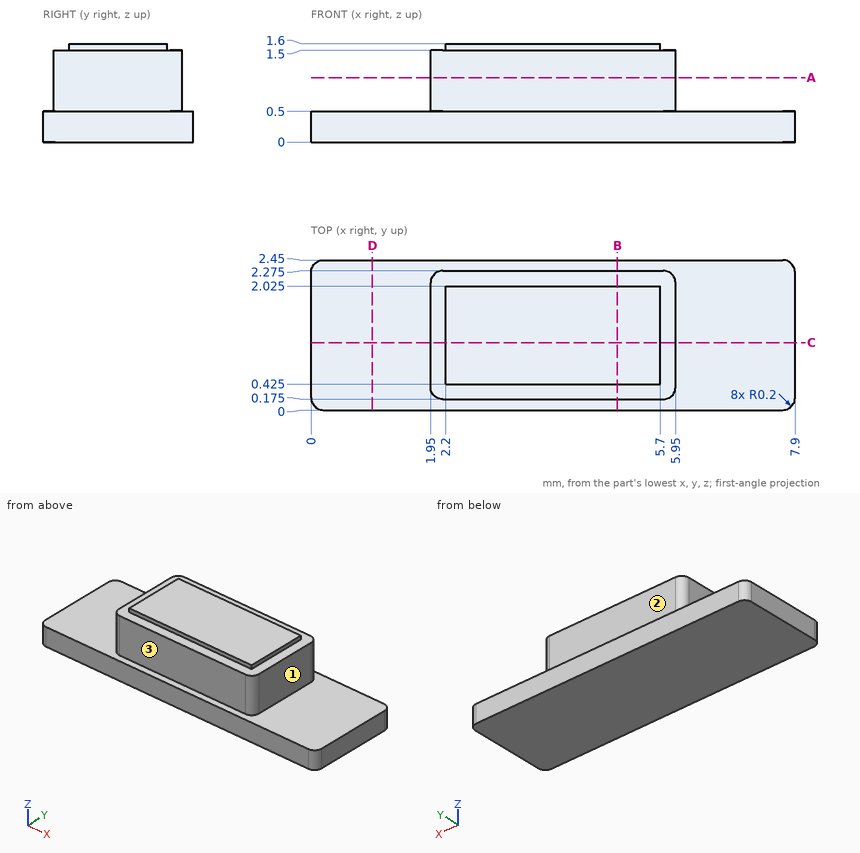
Input: dimensioned drawing with shaded views. Units: mm. Origin: part minimum x, y, z. A direction names the side the tool comes from. Round coordinates to 2 decimals unless told otherwise and drop trailing zeros. Order: outer loops, then holes, each group sorted by start corner. A loop starts at its lowest first (then second) coordinate and runs counter-clockwise, first axis right, second up. Notation, with made-up numbers: (24.25, 47) -> (34.25, 47) arc R33 ccw to (34.25, 78) -> close; hole circle Ø5 at (85.25, 19.5). An arc over 180 degrees is marked (long way). Put each result on its own line as item: value. Start each with the question number.
Q1. Section A-A on z = 1.05. Return the cut outline in (x, y) (3 decimals), and give its area (3 significant figures).
Q2. Line query: probe 1 along Z at (x, y) = (2, 1.35); probe 2 along Z at (x, y) = (7, 2); probe 3 along X at (y, z) = (0.55, 1.4). Output: solid intervals per line, ascending.
Q3. Reachability of the marked faces 1, 2 and 3 from +Z, -Z, +X, -X, +Y, -Y: full face, straight path, thin tool, end or side. Return the list, or none.
Q4. Section B-B on x = 5. Return the cut outline in (y, z) (3 decimals), and give its area (4 significant figures).
Q5. First-contact query: pin 1 (0.8 mm diameter, centred on x = 3, z = 1, fed in from -Y) (3 decimals); pin 2 (1 mm diameter, centred on x = 1, y = 1, fed in from +Z). Flat tips, straight axial feed; report the tip coordinate or a pass-through.
Q6. Section C-C on y = 1.1. Return the cut outline in (x, z).
Q7. Section D-D on x = 1. Return the cut outline in (y, z), and give its area (4 significant figures).
Ans:
1. outline: (1.95, 0.375) arc R0.2 ccw to (2.15, 0.175) -> (5.75, 0.175) arc R0.2 ccw to (5.95, 0.375) -> (5.95, 2.075) arc R0.2 ccw to (5.75, 2.275) -> (2.15, 2.275) arc R0.2 ccw to (1.95, 2.075) -> close
1. area: 8.37 mm2
2. probe 1: z = 0 to 1.5
2. probe 2: z = 0 to 0.5
2. probe 3: x = 1.95 to 5.95
3. face 1: +Z, +X, +Y, -Y
3. face 2: +Z, +X, -X, +Y
3. face 3: +Z, +X, -X, -Y
4. outline: (0, 0) -> (2.45, 0) -> (2.45, 0.5) -> (2.275, 0.5) -> (2.275, 1.5) -> (2.025, 1.5) -> (2.025, 1.6) -> (0.425, 1.6) -> (0.425, 1.5) -> (0.175, 1.5) -> (0.175, 0.5) -> (0, 0.5) -> close
4. area: 3.485 mm2
5. pin 1: stops at y = 0.175
5. pin 2: stops at z = 0.5
6. outline: (0, 0) -> (7.9, 0) -> (7.9, 0.5) -> (5.95, 0.5) -> (5.95, 1.5) -> (5.7, 1.5) -> (5.7, 1.6) -> (2.2, 1.6) -> (2.2, 1.5) -> (1.95, 1.5) -> (1.95, 0.5) -> (0, 0.5) -> close
7. outline: (0, 0) -> (2.45, 0) -> (2.45, 0.5) -> (0, 0.5) -> close
7. area: 1.225 mm2
